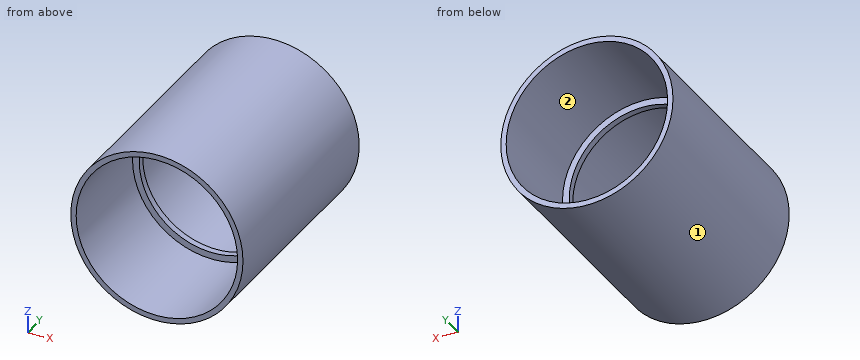
```python
from build123d import *

# Parameters (mm, degrees)
F0_R          = 40.64
F1_DEPTH      = 1.5875
F2_R          = 34.925
F3_DEPTH      = 1.5885
F3_DEPTH_BACK = 1.5885
F5_R          = 40.64
F6_DEPTH      = 50.8
F7_R          = 38.1
F8_DEPTH      = 50.8


with BuildPart() as f1:
    # F0 (on Front) → F1 (new body, symmetric)
    with BuildSketch(Plane.XZ):
        Circle(F0_R)
    extrude(amount=F1_DEPTH, both=True)

    # F2 (on Front) → F3 (cut, two sides)
    with BuildSketch(Plane.XZ) as f3_sk:
        Circle(F2_R)
    extrude(amount=F3_DEPTH, mode=Mode.SUBTRACT)
    extrude(f3_sk.sketch, amount=-F3_DEPTH_BACK, mode=Mode.SUBTRACT)

    # F5 (on offset) → F6 (join)
    with BuildSketch(Plane.XZ.offset(1.5875)):
        Circle(F5_R)
    extrude(amount=F6_DEPTH)

    # F7 (on face) → F8 (cut)
    with BuildSketch(Plane.XZ.offset(52.3875)):
        Circle(F7_R)
    extrude(amount=-F8_DEPTH, mode=Mode.SUBTRACT)

    # F9: F1 across plane


with BuildPart() as f1_1:
    add(f1.part)
    add(f1.part.mirror(Plane.XZ))


solid = f1_1.part
```
The listing builds one solid part. Answer for the finished solid, in the listing's coordinates (mm). Face numbers are marked on the shaded views. Give positions to 0.01 mm unless a question says otherwise; leave off trailing zeros. Order: outer loops, then holes, each group sorted by start corner. A loop starts at its lowest first (then second) coordinate and runs counter-clockwise, first axis right, second up. Notation, with made-up numbers: (-33.5, 9.25) - (-17.5, 9.25) arc R7 cw to (-17.5, 13.25) - close; hole circle Ø3 at (55.25, 79). An arc over 180 degrees is marked (long way). Use one line per item in the form item = value. Start each with the question number.
(1) Flat-ended cylindrical pins translate along their axes: pin 1 Ø6 at (y, z) = (13, 17.5) entering from +X; pin 2 Ø3 at (y, z) = (-11, 19) entering from +X; pin 3 Ø1.5 at (y, z) = (35.5, 13) entering from +X; pin 4 Ø23 at (x, z) = (0, -17) entering from -Y. Find the tip coordinate at first contact, or state that the pin passes through.
(2) A cutting plane is placed at C-C, the plane y = 3.5. Write down the section's boundary in (x, z), then the cut area to 3 significant figures.
(3) A cutting plane is placed at A-A, the plane x = 0. Write down the section's boundary in (y, z) (1 decimal).
(4) The mould has two halves that part along Z. Classify the marked faces 1 and 2: released by +Z, released by -Z, zero draft, split by the parting line, or undercut.
(5) A cutting plane is placed at B-B, the plane z = 0. Write down the section's boundary in (x, y) (1 decimal), then the cut area to 3 significant figures.
(6) Consider line 1 (Z direction, x = 0, y = -12); line 2 (Z direction, x = 0, y = 0.7) (3 decimals); line 3 (X direction, y = 29, z = 1). Determine where each line is inside the solid, lowest interval first. Write a range as from..to.
Ans:
q1.pin_1 = 37.97
q1.pin_2 = 36.68
q1.pin_3 = 38.75
q1.pin_4 = through
q2.outline = circle Ø81.28 at (0, 0); hole circle Ø76.2 at (0, 0)
q2.area = 628 mm^2
q3.outline = (-52.4, -40.6) - (52.4, -40.6) - (52.4, -38.1) - (1.6, -38.1) - (1.6, -34.9) - (-1.6, -34.9) - (-1.6, -38.1) - (-52.4, -38.1) - close; (-52.4, 38.1) - (-1.6, 38.1) - (-1.6, 34.9) - (1.6, 34.9) - (1.6, 38.1) - (52.4, 38.1) - (52.4, 40.6) - (-52.4, 40.6) - close
q4.face_1 = split by the parting line
q4.face_2 = undercut
q5.outline = (-40.6, -52.4) - (-38.1, -52.4) - (-38.1, -1.6) - (-34.9, -1.6) - (-34.9, 1.6) - (-38.1, 1.6) - (-38.1, 52.4) - (-40.6, 52.4) - close; (34.9, -1.6) - (38.1, -1.6) - (38.1, -52.4) - (40.6, -52.4) - (40.6, 52.4) - (38.1, 52.4) - (38.1, 1.6) - (34.9, 1.6) - close
q5.area = 552 mm^2
q6.line_1 = -40.64..-38.1, 38.1..40.64
q6.line_2 = -40.64..-34.925, 34.925..40.64
q6.line_3 = -40.63..-38.09, 38.09..40.63
